Can you work these out from the model? Positions are in its coordinate system, mm. A direction names the side the tool comes from. Coordinates: 2 decimals unless noted, no trailing zeros. Order: outer loops, then holes, each group sorted by start corner. A loop starts at its lowest first (then second) coordinate and runs counter-clockwise, first axis right, second up. Notation, with made-up numbers: (-12, 56.5) -> (43, 56.5) arc R26 ccw to (43, 81.5) -> close; hole circle Ø3 at (83.25, 53.25). An arc over 180 degrees is marked (long way). Write item = value, one per line.
```python
from build123d import *

# Parameters (mm, degrees)
SKETCH6_W     = 1.5113
SKETCH6_H     = 1.905
TOOL_RADIUS_R = 0.4064


with BuildPart() as part:
    # Sketch4 → Revolve1 (revolve)
    with BuildSketch(Plane(origin=(0, 0, 0), x_dir=(0, 0, -1), z_dir=(1, 0, 0)), mode=Mode.PRIVATE) as revolve1_sk:
        Polygon((34.2773, 0), (19.05, -21.746838143), (19.05, -38.149257502), (20.382233443, -46.030856842), (29.1846, -46.030856842), (29.1846, -25.050456842), (34.2773, -25.050456842), align=None)
    revolve(revolve1_sk.sketch.rotate(Axis((0, 0, 0), (0, -1, 0)), 180), axis=Axis((0, 0, 0), (0, -1, 0)))

    # Sketch6 → Spring Groove (revolve, cut)
    with BuildSketch(Plane(origin=(0, 0, 0), x_dir=(0, 0, -1), z_dir=(1, 0, 0)), mode=Mode.PRIVATE) as spring_groove_sk:
        with Locations((33.52165, -7.3025)):
            Rectangle(SKETCH6_W, SKETCH6_H)
    revolve(spring_groove_sk.sketch.rotate(Axis((0, 11.364369063, 0), (0, -1, 0)), 180), axis=Axis((0, 11.364369063, 0), (0, -1, 0)), mode=Mode.SUBTRACT)

    # Tool Radius
    tool_radius_edges = [part.edges().sort_by_distance(p)[0] for p in [
        (0, -6.35, -32.766),
        (0, -8.255, -32.766),
        (0, -46.030856842, -29.1846),
        (0, -25.050456842, -29.1846),
        (0, -25.050456842, -34.2773),
    ]]
    fillet(tool_radius_edges, radius=TOOL_RADIUS_R)


solid = part.part
```
Item 1: I want a section at C-C, the plane y = -17. Please give me the cut outline in (x, z).
A:
outline = circle Ø68.55 at (0, 0); hole circle Ø44.75 at (0, 0)
Item 2: If I drill on probe 1 along X at (y, z) = (-30.25, 0); probe 2 along Z at (x, y) = (25, -7); probe 3 along Z at (x, y) = (21.5, -2.5), over which ranges is the centre line in solid material (lowest first)?
A:
probe_1 = -29.18 to -19.05, 19.05 to 29.18
probe_2 = -21.18 to -15.43, 15.43 to 21.18
probe_3 = -26.7 to -24.41, 24.41 to 26.7
Item 3: I'm going to push flat-ended pins straight in: P1, Ø4, axis at y = -30.5, z = -27, coming from the -X side; P2, Ø5, axis at x = -25.5, y = -39.5, coming from the +Z side (3 decimals); P3, Ø6, axis at y = -8, z = 4, coming from the +X side. Where does each tip first touch, or does it pass through?
A:
P1 = -15.06
P2 = 17.965
P3 = 34.26
Item 4: If we mould it in two halves opening along X, with no side actions, what happens to faces 1 (the conical face through (18.678, -38.642, -4.148)), 2 (the flat face through (30, -25.05, 0)), 3 (the cylindrical face through (-9.842, -7.295, 31.253))? For each: pulls with the +X half, pulls with the -X half, needs draft (parallel to the pull), parting line crosses it, or undercut.
A:
face_1 = undercut
face_2 = needs draft
face_3 = parting line crosses it
Item 5: For faces 4 (the cylindrical face through (-19.724, -35.399, -21.51)), 5 (the flat face through (-20, -46.031, -6)), 6 (the flat face through (-28.09, -6.35, 17.93)), which set-ups out of +Z, -Z, +X, -X, +Y, -Y let a thin tool reach every point of the face, with its end or its side?
A:
face_4 = -Y
face_5 = +Z, -Z, +X, -X, -Y
face_6 = none
